from build123d import *

# Parameters (mm, degrees)
F0_R     = 12.7
F1_DEPTH = 508
F2_R     = 12.7
F3_T     = -3.175


with BuildPart() as f1:
    # F0 (on Front) → F1 (new body)
    with BuildSketch(Plane.XZ):
        Circle(F0_R)
    extrude(amount=-F1_DEPTH)

    # F2
    f2_edges = [f1.edges().sort_by_distance(p)[0] for p in [
        (-12.7, 508, 0),
    ]]
    fillet(f2_edges, radius=F2_R)

    # F3
    f3_openings = [f1.faces().sort_by_distance(p)[0] for p in [
        (0, 0, 0),
    ]]
    offset(amount=F3_T, openings=f3_openings)


solid = f1.part
Geometry: final body of the model. Coordinates: model frame, mm. Give positions to 0.01 mm unless a question says otherwise; leave off trailing zeros. Write each loop counter-clockwise with the first axis right and the second up, starting at its lowest first coordinate (ties: lowest second). Pieces come first, ordered by that corner, then holes.
(1) Cut plane B-B, the plane z = 0. Return loops of the section in (x, y) (3 decimals), then the cut area to 3 significant figures.
(2) Ray query, line 1 (Z direction, x = 0, y = 169.5) (3 decimals); line 2 (Z direction, x = -2.5, y = 188.5); line 3 (X direction, y = 449.5, z = 3). Return the intervals inside material, ascending.
(3) Cut plane A-A, the plane x = 0. Return loops of the section in (y, z) (3 decimals), then the cut area to 3 significant figures.
(4) Cut plane C-C, the plane y = 56. Return loops of the section in (x, z) (3 decimals).
(5) Mould query, pull axis X, two halves, no side actions, for faces 1 (the flat face through (5, 0, 9)), 2 (the cylindrical face through (-7.559, 244.183, -5.796)), 3 (the cylindrical face through (-2.75, 244.18, -12.4)). Classes: released by +X, released by -X, zero draft, split by the parting line, or undercut.
(6) First-contact query: P1, Ø6, axis at x = 1.5, z = 9, coming from the +Y side; P2, Ø4, axis at y = 341.5, z = -3.5, coming from the -X side; P3, Ø12, axis at y = 377.5, z = -10, coming from the +X side. Flat tips, straight axial feed; report the tip coordinate or a pass-through.
Values follow:
1. outline: (-12.7, 0) - (-9.525, 0) - (-9.525, 495.3) arc R9.525 cw to (9.525, 495.3) - (9.525, 0) - (12.7, 0) - (12.7, 495.3) arc R12.7 ccw to (-12.7, 495.3) - close
1. area: 3,260 mm2
2. line 1: z = -12.7 to -9.525, 9.525 to 12.7
2. line 2: z = -12.45 to -9.19, 9.19 to 12.45
2. line 3: x = -12.34 to -9.04, 9.04 to 12.34
3. outline: (0, -12.7) - (495.3, -12.7) arc R12.7 ccw to (495.3, 12.7) - (0, 12.7) - (0, 9.525) - (495.3, 9.525) arc R9.525 cw to (495.3, -9.525) - (0, -9.525) - close
3. area: 3,260 mm2
4. outline: circle Ø25.4 at (0, 0); hole circle Ø19.05 at (0, 0)
5. face 1: zero draft
5. face 2: undercut
5. face 3: split by the parting line
6. P1: stops at y = 506.43
6. P2: stops at x = -12.61
6. P3: stops at x = 12.05
